Build history of the part. All positions in model axes, mm. Face numbers are marked on the shaded views. Give positions to 0.01 mm unless a question says otherwise; leave off trailing zeros. Order: outer loops, then holes, each group sorted by start corner. A loop starts at its lowest first (then second) coordinate and runs counter-clockwise, first axis right, second up. Notation, with made-up numbers: (-39, 49) - (-10, 49) arc R19 cw to (-10, 68) - close; hole circle Ø9 at (50, 65.5). An arc over 180 degrees is marked (long way). Use a Markdown table: item, result.
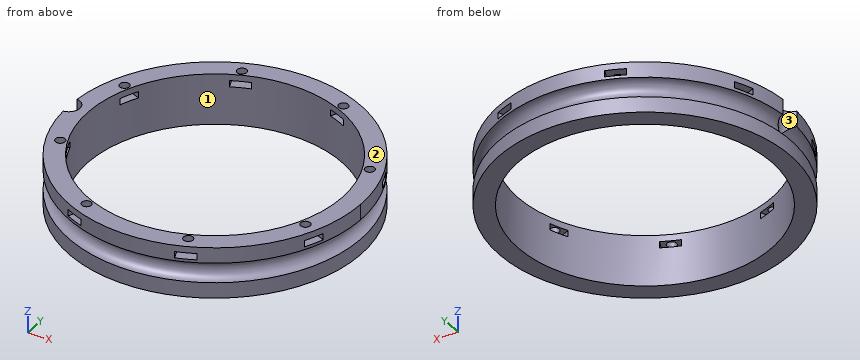
from build123d import *

# Parameters (mm, degrees)
BOX331_W                    = 6
BOX331_H                    = 8
BOX331_DEPTH                = 2
BOX331_PLACEMENT_ANGLE      = 45
BOX329_W                    = 6
BOX329_H                    = 8
BOX329_DEPTH                = 2
BOX328_W                    = 6
BOX328_H                    = 8
BOX328_DEPTH                = 2
BOX333_W                    = 6
BOX333_H                    = 8
BOX333_DEPTH                = 2
BOX333_PLACEMENT_ANGLE      = 135
BOX332_W                    = 6
BOX332_H                    = 8
BOX332_DEPTH                = 2
BOX327_W                    = 6
BOX327_H                    = 8
BOX327_DEPTH                = 2
BOX327_PLACEMENT_ANGLE      = 225
BOX330_W                    = 6
BOX330_H                    = 8
BOX330_DEPTH                = 2
BOX323_W                    = 6
BOX323_H                    = 8
BOX323_DEPTH                = 2
BOX323_PLACEMENT_ANGLE      = 45
COMPOUND696_PLACEMENT_ANGLE = 22.5
CYLINDER713_R               = 1.5
CYLINDER713_DEPTH           = 12
CYLINDER713_PLACEMENT_ANGLE = 45
CYLINDER712_R               = 1.5
CYLINDER712_DEPTH           = 12
CYLINDER711_R               = 1.5
CYLINDER711_DEPTH           = 12
CYLINDER711_PLACEMENT_ANGLE = 135
CYLINDER703_R               = 1.5
CYLINDER703_DEPTH           = 12
CYLINDER709_R               = 1.5
CYLINDER709_DEPTH           = 12
CYLINDER709_PLACEMENT_ANGLE = 225
CYLINDER710_R               = 1.5
CYLINDER710_DEPTH           = 12
CYLINDER698_R               = 1.5
CYLINDER698_DEPTH           = 12
CYLINDER698_PLACEMENT_ANGLE = 45
CYLINDER701_R               = 1.5
CYLINDER701_DEPTH           = 12
COMPOUND698_PLACEMENT_ANGLE = 22.5
CYLINDER694_R               = 3.5
CYLINDER694_DEPTH           = 20
TORUS006_R                  = 3.1
TUBE075_R                   = 46
TUBE075_R_2                 = 40
TUBE075_DEPTH               = 16


with BuildPart() as krychle331:
    # Box331 → Box331 (new body)
    with BuildSketch(Plane.XY):
        with Locations((3, 4)):
            Rectangle(BOX331_W, BOX331_H)
    extrude(amount=BOX331_DEPTH)


with BuildPart() as krychle331_1:
    # Box331 placement: moved
    add(krychle331.part.moved(Location((30.405592, -34.648232, 33))).rotate(Axis((30.405592, -34.648232, 33), (0, 0, 1)), BOX331_PLACEMENT_ANGLE))


with BuildPart() as krychle329:
    # Box329 → Box329 (new body)
    with BuildSketch(Plane(origin=(46, -3, 33), x_dir=(0, 1, 0), z_dir=(0, 0, 1))):
        with Locations((3, 4)):
            Rectangle(BOX329_W, BOX329_H)
    extrude(amount=BOX329_DEPTH)


with BuildPart() as krychle328:
    # Box328 → Box328 (new body)
    with BuildSketch(Plane(origin=(-3, -46, 33), x_dir=(1, 0, 0), z_dir=(0, 0, 1))):
        with Locations((3, 4)):
            Rectangle(BOX328_W, BOX328_H)
    extrude(amount=BOX328_DEPTH)


with BuildPart() as krychle333:
    # Box333 → Box333 (new body)
    with BuildSketch(Plane.XY):
        with Locations((3, 4)):
            Rectangle(BOX333_W, BOX333_H)
    extrude(amount=BOX333_DEPTH)


with BuildPart() as krychle333_1:
    # Box333 placement: moved
    add(krychle333.part.moved(Location((34.648232, 30.405592, 33))).rotate(Axis((34.648232, 30.405592, 33), (0, 0, 1)), BOX333_PLACEMENT_ANGLE))


with BuildPart() as krychle332:
    # Box332 → Box332 (new body)
    with BuildSketch(Plane(origin=(3, 46, 33), x_dir=(-1, 0, 0), z_dir=(0, 0, 1))):
        with Locations((3, 4)):
            Rectangle(BOX332_W, BOX332_H)
    extrude(amount=BOX332_DEPTH)


with BuildPart() as krychle327:
    # Box327 → Box327 (new body)
    with BuildSketch(Plane.XY):
        with Locations((3, 4)):
            Rectangle(BOX327_W, BOX327_H)
    extrude(amount=BOX327_DEPTH)


with BuildPart() as krychle327_1:
    # Box327 placement: moved
    add(krychle327.part.moved(Location((-30.405592, 34.648232, 33))).rotate(Axis((-30.405592, 34.648232, 33), (0, 0, 1)), BOX327_PLACEMENT_ANGLE))


with BuildPart() as krychle330:
    # Box330 → Box330 (new body)
    with BuildSketch(Plane(origin=(-46, 3, 33), x_dir=(0, -1, 0), z_dir=(0, 0, 1))):
        with Locations((3, 4)):
            Rectangle(BOX330_W, BOX330_H)
    extrude(amount=BOX330_DEPTH)


with BuildPart() as compound696:
    # Box323 → Box323 (new body)
    with BuildSketch(Plane.XY):
        with Locations((3, 4)):
            Rectangle(BOX323_W, BOX323_H)
    extrude(amount=BOX323_DEPTH)


with BuildPart() as compound696_1:
    # Box323 placement: moved
    add(compound696.part.moved(Location((-34.648232, -30.405592, 33))).rotate(Axis((-34.648232, -30.405592, 33), (0, 0, -1)), BOX323_PLACEMENT_ANGLE))

    # Compound696: union Krychle331, Krychle329, Krychle328, Krychle333, Krychle332, Krychle327, Krychle330
    add(krychle331_1.part)
    add(krychle329.part)
    add(krychle328.part)
    add(krychle333_1.part)
    add(krychle332.part)
    add(krychle327_1.part)
    add(krychle330.part)


with BuildPart() as compound696_2:
    # Compound696 placement: moved
    add(compound696_1.part.rotate(Axis((0, 0, 0), (0, 0, 1)), COMPOUND696_PLACEMENT_ANGLE))


with BuildPart() as obj1:
    # Cylinder713 → Cylinder713 (new body)
    with BuildSketch(Plane.XY):
        Circle(CYLINDER713_R)
    extrude(amount=CYLINDER713_DEPTH)


with BuildPart() as obj1_1:
    # Cylinder713 placement: moved
    add(obj1.part.moved(Location((29.698485, -29.698485, 33.5))).rotate(Axis((29.698485, -29.698485, 33.5), (0, 0, 1)), CYLINDER713_PLACEMENT_ANGLE))


with BuildPart() as obj2:
    # Cylinder712 → Cylinder712 (new body)
    with BuildSketch(Plane(origin=(42, 0, 33.5), x_dir=(0, 1, 0), z_dir=(0, 0, 1))):
        Circle(CYLINDER712_R)
    extrude(amount=CYLINDER712_DEPTH)


with BuildPart() as obj3:
    # Cylinder711 → Cylinder711 (new body)
    with BuildSketch(Plane.XY):
        Circle(CYLINDER711_R)
    extrude(amount=CYLINDER711_DEPTH)


with BuildPart() as obj3_1:
    # Cylinder711 placement: moved
    add(obj3.part.moved(Location((29.698485, 29.698485, 33.5))).rotate(Axis((29.698485, 29.698485, 33.5), (0, 0, 1)), CYLINDER711_PLACEMENT_ANGLE))


with BuildPart() as obj4:
    # Cylinder703 → Cylinder703 (new body)
    with BuildSketch(Plane(origin=(0, 42, 33.5), x_dir=(-1, 0, 0), z_dir=(0, 0, 1))):
        Circle(CYLINDER703_R)
    extrude(amount=CYLINDER703_DEPTH)


with BuildPart() as obj5:
    # Cylinder709 → Cylinder709 (new body)
    with BuildSketch(Plane.XY):
        Circle(CYLINDER709_R)
    extrude(amount=CYLINDER709_DEPTH)


with BuildPart() as obj5_1:
    # Cylinder709 placement: moved
    add(obj5.part.moved(Location((-29.698485, 29.698485, 33.5))).rotate(Axis((-29.698485, 29.698485, 33.5), (0, 0, 1)), CYLINDER709_PLACEMENT_ANGLE))


with BuildPart() as obj6:
    # Cylinder710 → Cylinder710 (new body)
    with BuildSketch(Plane(origin=(-42, 0, 33.5), x_dir=(0, -1, 0), z_dir=(0, 0, 1))):
        Circle(CYLINDER710_R)
    extrude(amount=CYLINDER710_DEPTH)


with BuildPart() as obj7:
    # Cylinder698 → Cylinder698 (new body)
    with BuildSketch(Plane.XY):
        Circle(CYLINDER698_R)
    extrude(amount=CYLINDER698_DEPTH)


with BuildPart() as obj7_1:
    # Cylinder698 placement: moved
    add(obj7.part.moved(Location((-29.698485, -29.698485, 33.5))).rotate(Axis((-29.698485, -29.698485, 33.5), (0, 0, -1)), CYLINDER698_PLACEMENT_ANGLE))


with BuildPart() as compound698:
    # Cylinder701 → Cylinder701 (new body)
    with BuildSketch(Plane(origin=(0, -42, 33.5), x_dir=(1, 0, 0), z_dir=(0, 0, 1))):
        Circle(CYLINDER701_R)
    extrude(amount=CYLINDER701_DEPTH)

    # Compound698: union obj1, obj2, obj3, obj4, obj5, obj6, obj7
    add(obj1_1.part)
    add(obj2.part)
    add(obj3_1.part)
    add(obj4.part)
    add(obj5_1.part)
    add(obj6.part)
    add(obj7_1.part)


with BuildPart() as compound698_1:
    # Compound698 placement: moved
    add(compound698.part.rotate(Axis((0, 0, 0), (0, 0, 1)), COMPOUND698_PLACEMENT_ANGLE))


with BuildPart() as obj8:
    # Cylinder694 → Cylinder694 (new body)
    with BuildSketch(Plane(origin=(-46.3, 0, 29), x_dir=(1, 0, 0), z_dir=(0, 0, 1))):
        Circle(CYLINDER694_R)
    extrude(amount=CYLINDER694_DEPTH)


with BuildPart() as obj9:
    # Torus006 → Torus006 (revolve)
    with BuildSketch(Plane(origin=(0, 0, 29), x_dir=(1, 0, 0), z_dir=(0, -1, 0))):
        with Locations((46, 0)):
            Circle(TORUS006_R)
    revolve(axis=Axis((0, 0, 29), (0, 0, 1)))


with BuildPart() as cut329:
    # Tube075 → Tube075 (new body)
    with BuildSketch(Plane.XY.offset(21)):
        Circle(TUBE075_R)
        Circle(TUBE075_R_2, mode=Mode.SUBTRACT)
    extrude(amount=TUBE075_DEPTH)

    # Cut325: cut obj9
    add(obj9.part, mode=Mode.SUBTRACT)

    # Cut326: cut obj8
    add(obj8.part, mode=Mode.SUBTRACT)

    # Cut328: cut Compound698
    add(compound698_1.part, mode=Mode.SUBTRACT)

    # Cut329: cut Compound696
    add(compound696_2.part, mode=Mode.SUBTRACT)


solid = cut329.part
1) Two-plate mould, pull along X, no slides. Class the marked faces 1, 2 and 3: +X half, -X half, draft (parallel to the pull), parting line (faces both ways), or undercut.
Computed:
| item | result |
|---|---|
| face 1 | undercut |
| face 2 | draft |
| face 3 | -X half |
2) Pin check, flat tips, straight feed: P1, Ø1.5, axis at y = 26.5, z = 34.5, coming from the +X side; P2, Ø1, axis at x = 10, z = 27, coming from the +Y side; P3, Ø2.5, axis at x = -38.8, y = 16.07, coming from the +Z side. Stop position of each tip, or through.
Computed:
| item | result |
|---|---|
| P1 | stops at x = 38.12 |
| P2 | stops at y = 43.03 |
| P3 | stops at z = 33 |
3) Wall check: line 1 (Y direction, x = -0.5, z = 32.75); line 2 (X direction, y = 18.5, z = 36); line 3 (Y direction, x = 28.5, z = 25.5). Give the ranges that are in metal, low to high. Write a range as from..to.
Computed:
| item | result |
|---|---|
| line 1 | y = -46..-40, 40..46 |
| line 2 | x = -42.12..-35.46, 35.46..42.12 |
| line 3 | y = -36.11..-28.07, 28.07..36.11 |
4) Slice it at A-A (x = 0). Write the cut outline in (y, z), and give its area (3 significant figures).
Computed:
| item | result |
|---|---|
| outline | (-46, 21) - (-40, 21) - (-40, 37) - (-46, 37) - (-46, 32.1) arc R3.1 cw to (-46, 25.9) - close; (40, 21) - (46, 21) - (46, 25.9) arc R3.1 cw to (46, 32.1) - (46, 37) - (40, 37) - close |
| area | 162 mm² |
5) Slice it at B-B (z = 23.25). Write the cut outline in (x, y), and give its area (3 significant figures).
Computed:
| item | result |
|---|---|
| outline | circle Ø92 at (0, 0); hole circle Ø80 at (0, 0) |
| area | 1,620 mm² |
